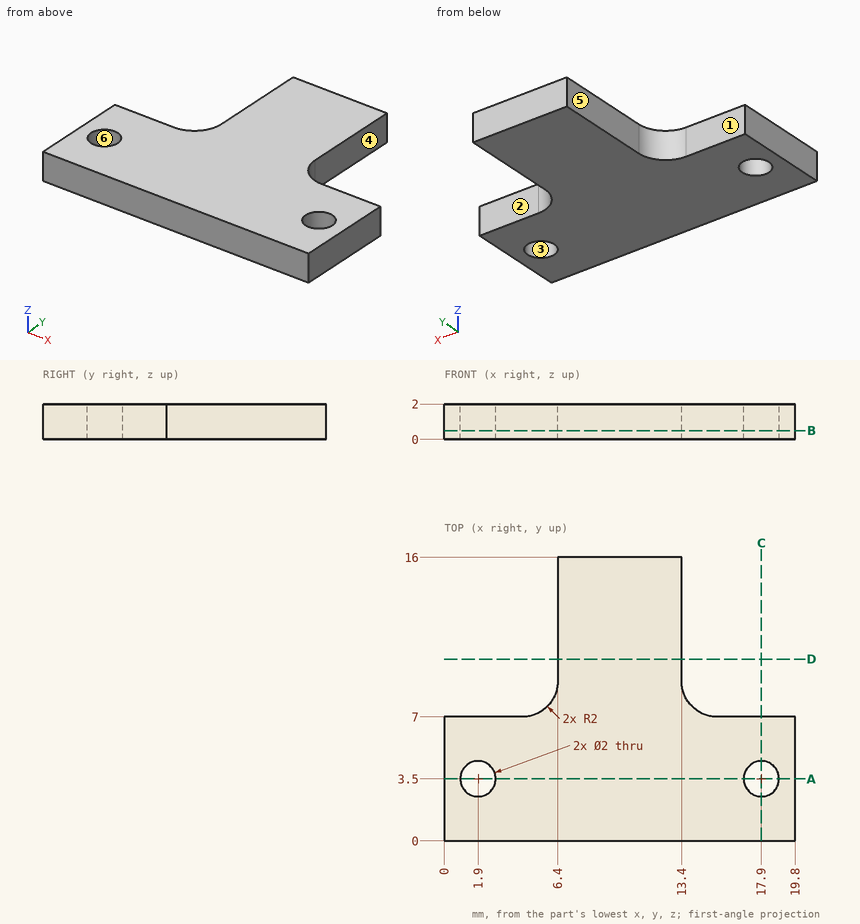
Source: three-view drawing plus pictorial views. Frame: mm from the lowest corner of the part. A direction names the side the tool comes from. Coordinates: 2 decimals unless noted, no trailing zeros. Loops run counter-clockwise (first coordinate to the right, second up) from the corner with the lowest first, then second, coordinate; pieces in that order, holes last. Notation, with made-up numbers: (24, 10) -> (50, 10) arc R21 cw to (50, 36) -> close; hole circle Ø9 at (26.25, -6.75). An arc over 180 degrees is marked (long way). Write each question's results on one line, items separated by ' | '. Start each with the question number.
Q1. Pull-direction query (X, two-part tool) for the marked faces 4, 5 and 6; classes: released by +X, released by -X, zero draft, split by the parting line, or undercut.
Q2. Section C-C, the plane x = 17.9. Return the cut outline in (y, z), plus the area to 3 significant figures.
Q3. Reachability of the marked faces 1, 2 and 3 from +Z, -Z, +X, -X, +Y, -Y: full face, straight path, thin tool, end or side. Return the list, or none.
Q4. Section D-D, the plane y = 10.25. Return the cut outline in (x, z).
Q5. Ray query, line 1 (Y direction, x = 1.9, z = 0.6); line 2 (X direction, y = 14.5, z = 1.65); line 3 (X direction, y = 2.75, z = 0.65). Return the intervals inside material, ascending. Write a range as from..to.
Q6. Section A-A, the plane y = 3.5. Return the cut outline in (x, z).
Q7. Pin query (flat end, axial travel): pin 1 (1 mm diameter, centred on x = 17.5, z = 1.5, fed in from +Y); pin 2 (0.6 mm diameter, centred on y = 12.5, z = 0.5, fed in from +X); pin 3 (1.8 mm diameter, centred on x = 17.9, y = 3.5, fed in from -Z). Return the tip coordinate at first contact, or that it passes through.
Q8. Section B-B, the plane z = 0.5. Return the cut outline in (x, y).
Found:
1) face 4: released by +X | face 5: released by -X | face 6: undercut
2) outline: (0, 0) -> (2.5, 0) -> (2.5, 2) -> (0, 2) -> close; (4.5, 0) -> (7, 0) -> (7, 2) -> (4.5, 2) -> close | area: 10.0 mm2
3) face 1: +Z, -Z, -X, +Y | face 2: +Z, -Z, +X, +Y | face 3: +Z, -Z
4) outline: (6.4, 0) -> (13.4, 0) -> (13.4, 2) -> (6.4, 2) -> close
5) line 1: 0..2.5, 4.5..7 | line 2: 6.4..13.4 | line 3: 0..1.24, 2.56..17.24, 18.56..19.8
6) outline: (0, 0) -> (0.9, 0) -> (0.9, 2) -> (0, 2) -> close; (2.9, 0) -> (16.9, 0) -> (16.9, 2) -> (2.9, 2) -> close; (18.9, 0) -> (19.8, 0) -> (19.8, 2) -> (18.9, 2) -> close
7) pin 1: y = 7 | pin 2: x = 13.4 | pin 3: through
8) outline: (0, 0) -> (19.8, 0) -> (19.8, 7) -> (15.4, 7) arc R2 cw to (13.4, 9) -> (13.4, 16) -> (6.4, 16) -> (6.4, 9) arc R2 cw to (4.4, 7) -> (0, 7) -> close; hole circle Ø2 at (1.9, 3.5); hole circle Ø2 at (17.9, 3.5)
